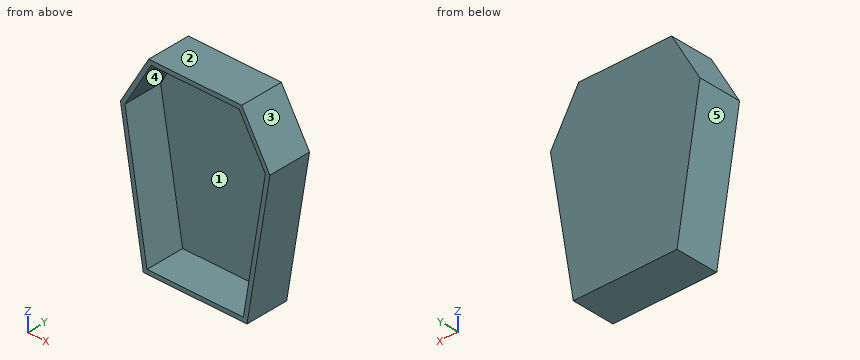
```python
from build123d import *

# Parameters (mm, degrees)
F2_DEPTH = 25.4
F3_T     = -2.54


with BuildPart() as f2:
    # F0 (on Front) → F2 (new body)
    with BuildSketch(Plane.XZ):
        Polygon((27.629351, 55.258706), (-27.341546, 55.258706), (-44.03428, 26.478129), (-30.50741, -56.122124), (30.795213, -56.122124), (44.322088, 26.478129), align=None)
    extrude(amount=-F2_DEPTH)

    # F3
    f3_openings = [f2.faces().sort_by_distance(p)[0] for p in [
        (0.143903, 0, 0.698193),
    ]]
    offset(amount=F3_T, openings=f3_openings)


solid = f2.part
```
Geometry: final body of the model. Coordinates: model frame, mm. Face numbers are marked on the shaded views. A direction names the side the tool comes from. Round coordinates to 2 decimals unless told otherwise and drop trailing zeros. Order: outer loops, then holes, each group sorted by start corner. A loop starts at its lowest first (then second) coordinate and runs counter-clockwise, first axis right, second up. Notation, with made-up numbers: (25.25, 14.25) -> (73.25, 14.25) arc R22 ccw to (73.25, 51.25) -> close; hole circle Ø10 at (-5, 8.5). An arc over 180 degrees is marked (long way). Use one line per item in the form item = value.
(1) Ray query, probe 1 along Z at (x, y) = (12.5, 1); probe 2 along Y at (x, z) = (36, 4.5); probe 3 along X at (y, z) = (2.25, 21). Return the intervals inside material, ascending. Write a range as [from, to].
Results list:
probe_1 = [-56.12, -53.58], [52.72, 55.26]
probe_2 = [22.86, 25.4]
probe_3 = [-43.14, -40.56], [40.85, 43.42]
(2) Draft query along X for the marked faces 1, 2 and 3. Return one class per face: pulls with the +X half, pulls with the -X half, needs draft (parallel to the pull), parting line crosses it, or undercut.
Results list:
face_1 = undercut
face_2 = needs draft
face_3 = pulls with the +X half
(3) First-contact query: pin 1 Ø10 at (x, z) = (-11.5, 27.5) entering from -Y. Flat tip, straight axial feed; report the tip coordinate or a pass-through.
Results list:
pin_1 = 22.86
(4) Section A-A on y = 11. Return loops of the section in (x, z), and give its area (3 significant figures).
Results list:
outline = (-44.03, 26.48) -> (-30.51, -56.12) -> (30.8, -56.12) -> (44.32, 26.48) -> (27.63, 55.26) -> (-27.34, 55.26) -> close; hole (-41.38, 25.99) -> (-28.35, -53.58) -> (28.64, -53.58) -> (41.67, 25.99) -> (26.17, 52.72) -> (-25.88, 52.72) -> close
area = 867 mm^2
(5) Section C-C on z = 8. Return loops of the section in (x, y), and give its area (3 significant figures).
Results list:
outline = (-41.01, 0) -> (-38.43, 0) -> (-38.43, 22.86) -> (38.72, 22.86) -> (38.72, 0) -> (41.3, 0) -> (41.3, 25.4) -> (-41.01, 25.4) -> close
area = 327 mm^2
(6) Access query for the marked faces 4 and 5. Directions: +Z, -Z, +X, -X, +Y, -Y. A direction counts if a zero-diameter tool reaches every point of the face in a straight line with its end or side. Return the directions, or none.
Results list:
face_4 = -Y
face_5 = -Z, -X, +Y, -Y
(7) Section B-B on x = 11.5. Return loops of the section in (y, z), and give its area (3 significant figures).
Results list:
outline = (0, -56.12) -> (25.4, -56.12) -> (25.4, 55.26) -> (0, 55.26) -> (0, 52.72) -> (22.86, 52.72) -> (22.86, -53.58) -> (0, -53.58) -> close
area = 399 mm^2
